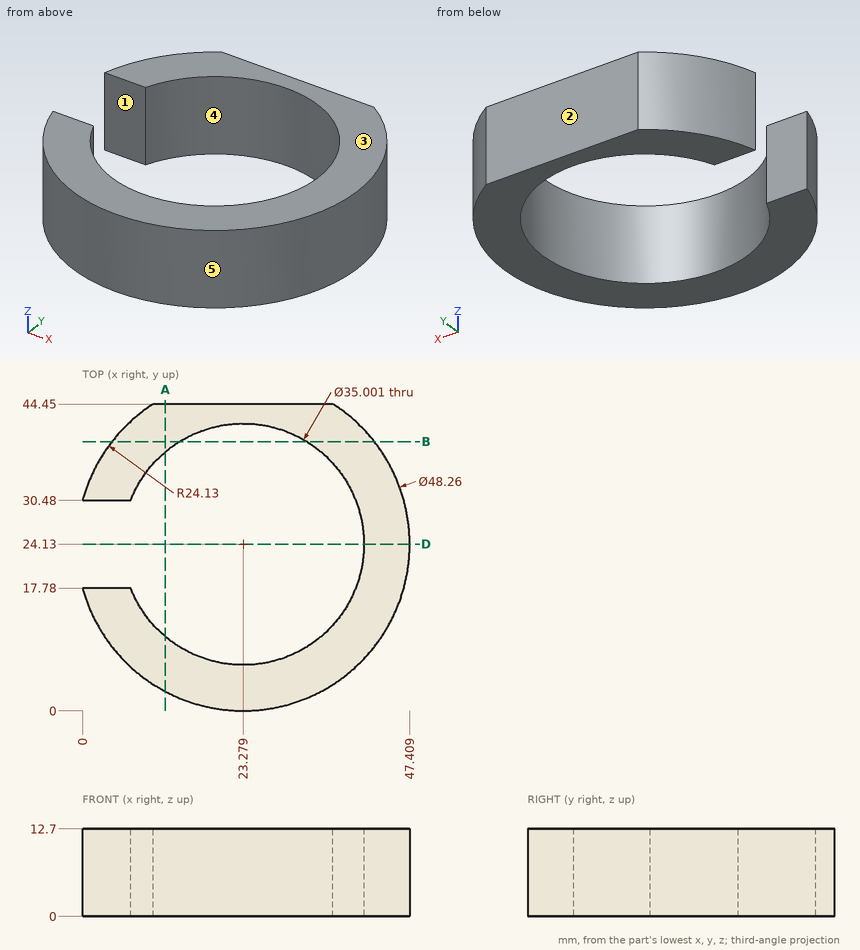
Verification items for this drawing (mm, ordinates from the low corner). A direction names the side the tool comes from. Round coordinates to 2 decimals unless told otherwise and drop trailing zeros. Order: outer loops, then holes, each group sorted by start corner. A loop starts at its lowest first (then second) coordinate and runs counter-clockwise, first axis right, second up. Notation, with made-up numbers: (-9, 87) - (19, 87) arc R15 cw to (19, 96) - close; hole circle Ø1 at (48, -26). An arc over 180 degrees is marked (long way). Use CSV: the item, a comma, the result in double quotes.
(1) Access from +Z, -Z, +X, -X, +Y, -Y to the whole of each face (thin tool, end or side, straight path). Record for the marked faces 1 and 2.
Entries:
face 1,"+Z, -Z, -X"
face 2,"+Z, -Z, +X, -X, +Y"
(2) Gauge pin test, flat ends, axial feed: pin 1 Ø4 at (x, y) = (5.5, 27.5) entering from -Z; pin 2 Ø5.5 at (x, z) = (3.5, 5) entering from -Y (1 decimal); pin 3 Ø2 at (x, z) = (5, 9) entering from +Y; pin 4 Ø1 at (y, z) = (36, 5) entering from -X (1 decimal). Record the tip position at first contact, or that the pin passes through.
Entries:
pin 1,"through"
pin 2,"y = 7"
pin 3,"y = 40.97"
pin 4,"x = 2"
(3) Section check A-A on x = 12. Record the boundary of the cut face in (y, z), and give its area (3 significant figures).
Entries:
outline,"(2.8, 0) - (10.75, 0) - (10.75, 12.7) - (2.8, 12.7) - close; (37.51, 0) - (44.45, 0) - (44.45, 12.7) - (37.51, 12.7) - close"
area,"189 mm^2"
(4) Section check D-D on y = 24.13. Record the boundary of the cut face in (x, z).
Entries:
outline,"(40.78, 0) - (47.41, 0) - (47.41, 12.7) - (40.78, 12.7) - close"
(5) Mould release check, pull along X, two halves, no side actions. Record for the marked faces 3, 4 and 5: released by +X, released by -X, zero draft, split by the parting line, or undercut.
Entries:
face 3,"zero draft"
face 4,"undercut"
face 5,"split by the parting line"
(6) Section check B-B on y = 39. Record the boundary of the cut face in (x, z) (1 decimal), and give its area (3 significant figures).
Entries:
outline,"(4.3, 0) - (14.1, 0) - (14.1, 12.7) - (4.3, 12.7) - close; (32.5, 0) - (42.3, 0) - (42.3, 12.7) - (32.5, 12.7) - close"
area,"248 mm^2"
(7) Thickness scan on probe 1 along Y at (x, z) = (23.5, 7); probe 2 along X at (y, z) = (36, 10); probe 3 along X at (y, z) = (24.13, 5.5). Record the ranges inside material, lowest first. Write a range as from..to.
Entries:
probe 1,"0..6.63, 41.63..44.45"
probe 2,"2.27..10.42, 36.14..44.29"
probe 3,"40.78..47.41"
